Job drawing, mm, ordinate dimensions from the low corner. One solid piece. Coordinates: 2 decimals unless noted, no trailing zeros. Write each loop counter-clockwise with the first axis right and the second up, starting at its lowest first coordinate (ties: lowest second). Pieces come first, ordered by that corner, then holes. Notation, with made-up numbers: (-2, -4.5) - (22, -4.5) arc R21 ccw to (22, 28.5) - close; hole circle Ø10 at (84, 71). An arc over 180 degrees is marked (long way). Use a Markdown table: item, result.
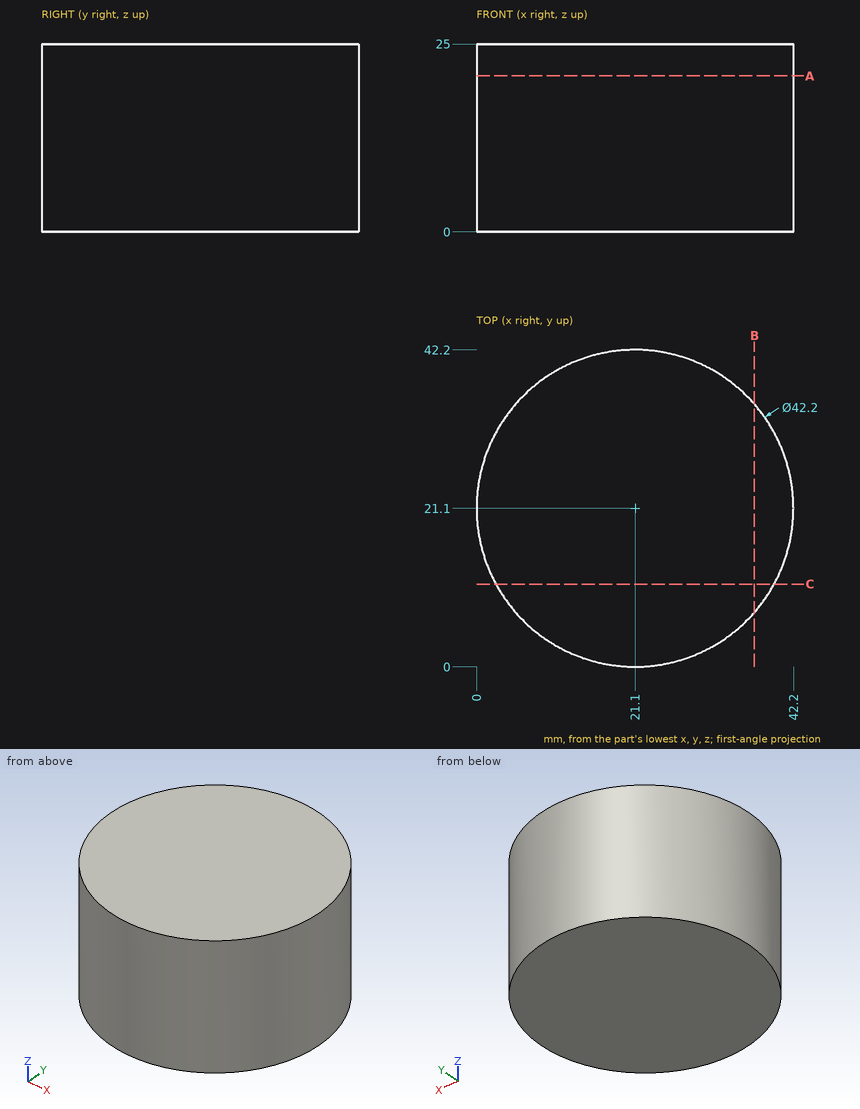
Item 1: Drill centre lines: probe 1 along X at (y, z) = (16, 23); probe 2 along Y at (x, z) = (30, 9); probe 3 along Y at (x, z) = (11, 16.5). Where is each one in solid material? Low to high.
From the geometry:
| item | result |
|---|---|
| probe 1 | 0.63 to 41.57 |
| probe 2 | 1.97 to 40.23 |
| probe 3 | 2.57 to 39.63 |
Item 2: Band-saw the part on B-B, the plane x = 37. Give the cut face in (y, z).
From the geometry:
| item | result |
|---|---|
| outline | (7.23, 0) - (34.97, 0) - (34.97, 25) - (7.23, 25) - close |
Item 3: Drop flat-ended pins along their axis: P1, Ø1, axis at x = 19, z = 22.5, coming from the -Y side; P2, Ø6, axis at y = 17.5, z = 7, coming from the +X side; P3, Ø1, axis at y = 6, z = 3, coming from the +X side. Give the stop position or say it passes through.
From the geometry:
| item | result |
|---|---|
| P1 | y = 0.06 |
| P2 | x = 42.19 |
| P3 | x = 36.33 |
Item 4: Band-saw the part on A-A, the plane z = 20.75. Give the cut face in (x, y).
From the geometry:
| item | result |
|---|---|
| outline | circle Ø42.2 at (21.1, 21.1) |
Item 5: Band-saw the part on C-C, the plane y = 11. Give the cut face in (x, z), then the cut area to 3 significant figures.
From the geometry:
| item | result |
|---|---|
| outline | (2.57, 0) - (39.63, 0) - (39.63, 25) - (2.57, 25) - close |
| area | 926 mm^2 |
